from build123d import *

# Parameters (mm, degrees)
SKETCH1_W           = 96
SKETCH1_H           = 68
BOSS_EXTRUDE1_DEPTH = 30
CUT_EXTRUDE1_DEPTH  = 69
SKETCH3_W           = 40
SKETCH3_H           = 10
CUT_EXTRUDE2_DEPTH  = 3
SKETCH4_W           = 12
SKETCH4_H           = 1
BOSS_EXTRUDE2_DEPTH = 5
SKETCH5_R           = 2.8
SKETCH5_R_2         = 1.5
CUT_EXTRUDE3_DEPTH  = 2.2
SKETCH5_2_R         = 1.5
CUT_EXTRUDE4_DEPTH  = 10


with BuildPart() as part:
    # Sketch1 → Boss-Extrude1 (new body)
    with BuildSketch(Plane(origin=(0, 0, 0), x_dir=(1, 0, 0), z_dir=(0, 1, 0))):
        Rectangle(SKETCH1_W, SKETCH1_H)
    extrude(amount=BOSS_EXTRUDE1_DEPTH)

    # Sketch2 → Cut-Extrude1 (cut, through all)
    with BuildSketch(Plane.XY.offset(34)):
        with BuildLine():
            Line((-48, 27), (-48, 41.348675948))
            Line((-48, 41.348675948), (48, 41.348675948))
            Line((48, 41.348675948), (48, 27))
            ThreePointArc((48, 27), (0, 30), (-48, 27))
        make_face()
    extrude(amount=-CUT_EXTRUDE1_DEPTH, mode=Mode.SUBTRACT)

    # Sketch3 → Cut-Extrude2 (cut)
    with BuildSketch(Plane.XY.offset(34)):
        with Locations((-23, 8)):
            Rectangle(SKETCH3_W, SKETCH3_H)
    extrude(amount=-CUT_EXTRUDE2_DEPTH, mode=Mode.SUBTRACT)

    # Sketch4 → Boss-Extrude2 (add)
    with BuildSketch(Plane(origin=(48, 0, 0), x_dir=(0, 0, -1), z_dir=(1, 0, 0))):
        with Locations((-20, 18.5)):
            Rectangle(SKETCH4_W, SKETCH4_H)
    extrude(amount=BOSS_EXTRUDE2_DEPTH)

    # Sketch5 → Cut-Extrude3 (cut)
    with BuildSketch(Plane.XZ):
        with Locations((-38, 24)):
            Circle(SKETCH5_R)
        with Locations((-38, 24)):
            Circle(SKETCH5_R_2, mode=Mode.SUBTRACT)
        with Locations((20, 24)):
            Circle(SKETCH5_R)
        with Locations((20, 24)):
            Circle(SKETCH5_R_2, mode=Mode.SUBTRACT)
        with Locations((20, -25)):
            Circle(SKETCH5_R)
        with Locations((20, -25)):
            Circle(SKETCH5_R_2, mode=Mode.SUBTRACT)
        with Locations((-38, -25)):
            Circle(SKETCH5_R)
        with Locations((-38, -25)):
            Circle(SKETCH5_R_2, mode=Mode.SUBTRACT)
    extrude(amount=-CUT_EXTRUDE3_DEPTH, mode=Mode.SUBTRACT)

    # Sketch5_2 → Cut-Extrude4 (cut)
    with BuildSketch(Plane.XZ):
        with Locations((-38, 24)):
            Circle(SKETCH5_2_R)
        with Locations((20, 24)):
            Circle(SKETCH5_2_R)
        with Locations((-38, -25)):
            Circle(SKETCH5_2_R)
        with Locations((20, -25)):
            Circle(SKETCH5_2_R)
    extrude(amount=-CUT_EXTRUDE4_DEPTH, mode=Mode.SUBTRACT)


solid = part.part
For this review, take the finished solid that the model builds, in its own axes (mm). A direction names the side the tool comes from. Round coordinates to 2 decimals unless told otherwise and drop trailing zeros. Write each loop counter-clockwise with the first axis right and the second up, starting at its lowest first coordinate (ties: lowest second). Pieces come first, ordered by that corner, then holes. Notation, with made-up numbers: M 39,49 L 76,49 A18 cw 76,84 Z; hole C 71.25,89.5 d3. An arc over 180 degrees is marked long. Write item = value, one per line. Start each with the question number.
(1) We need section D-D (z = 16). Give the boundary of the cut face in (x, y), then the cut area to 3 significant figures.
(2) The part is to be moulded in two halves that separate along X. For faces 1 (the face through (-1, 0, 0)), 2 (the face through (-48, 13, 0)), 3 (the face through (-40.064, 1.085, -23.108)), say which applies: +X half, -X half, draft (parallel to the pull), parting line (faces both ways), or undercut.
(3) We need section A-A (z = 24). Give the boundary of the cut face in (x, y).
(4) Clearance check with flat-ended pins moving along their axes: pin 1 Ø8 at (x, z) = (20, -19.5) entering from -Y; pin 2 Ø1.8 at (x, z) = (-38, -25) entering from -Y; pin 3 Ø3.5 at (x, z) = (20.5, 23.5) entering from -Y; pin 4 Ø2.5 at (x, z) = (20, 24) entering from +Y. State where each tip first meets the part, or that it passes through.
(5) For faces 4 (the face through (21.2, 2.2, 22.8)), 5 (the face through (50, 18, 20)), 6 (the face through (-23, 8, 31)), list the 3-axis set-ups (+Z, -Z, +X, -X, +Y, -Y) from which the entire face can be reached by the end or side of a thin tool; tool diameter is ignored.
(6) We need section B-B (y = 4.5). Give the boundary of the cut face in (x, z).
(7) For line 1 along Z through (x, y) = (20, 0.7); line 2 along X through (y, z) = (9.75, 6); line 3 along Y through (x, z) = (-1.5, -6.5), list the stretches that pass through material, from the lowest coordinate up.
(8) We need section C-C (x = -38). Give the boundary of the cut face in (y, z), then the cut area to 3 significant figures.
Results found:
q1.outline = M -48,0 L 48,0 L 48,18 L 53,18 L 53,19 L 48,19 L 48,27 A385.5 ccw -48,27 Z
q1.area = 2,790 mm²
q2.face_1 = draft
q2.face_2 = -X half
q2.face_3 = undercut
q3.outline = M -48,0 L -40.8,0 L -40.8,2.2 L -39.5,2.2 L -39.5,10 L -36.5,10 L -36.5,2.2 L -35.2,2.2 L -35.2,0 L 17.2,0 L 17.2,2.2 L 18.5,2.2 L 18.5,10 L 21.5,10 L 21.5,2.2 L 22.8,2.2 L 22.8,0 L 48,0 L 48,18 L 53,18 L 53,19 L 48,19 L 48,27 A385.5 ccw -48,27 Z
q4.pin_1 = 0
q4.pin_2 = 10
q4.pin_3 = 2.2
q4.pin_4 = 29.54
q5.face_4 = -Y
q5.face_5 = +Z, -Z, +X, -Y
q5.face_6 = +Z
q6.outline = M -48,-34 L 48,-34 L 48,34 L -3,34 L -3,31 L -43,31 L -43,34 L -48,34 Z; hole C -38,-25 d3; hole C -38,24 d3; hole C 20,-25 d3; hole C 20,24 d3
q7.line_1 = -34 to -27.8, -22.2 to 21.2, 26.8 to 34
q7.line_2 = -48 to 48
q7.line_3 = 0 to 30
q8.outline = M 0,-34 L 28.12,-34 L 28.12,34 L 13,34 L 13,31 L 3,31 L 3,34 L 0,34 L 0,26.8 L 2.2,26.8 L 2.2,25.5 L 10,25.5 L 10,22.5 L 2.2,22.5 L 2.2,21.2 L 0,21.2 L 0,-22.2 L 2.2,-22.2 L 2.2,-23.5 L 10,-23.5 L 10,-26.5 L 2.2,-26.5 L 2.2,-27.8 L 0,-27.8 Z
q8.area = 1,810 mm²
